Build history of the part. All positions in model axes, mm. A direction names the side the tool comes from. Round coordinates to 2 decimals unless told otherwise and drop trailing zeros. Write each loop counter-clockwise with the first axis right and the second up, starting at its lowest first coordinate (ties: lowest second). Pieces come first, ordered by that corner, then holes. Notation, with made-up numbers: M -14,-23 L 7,-23 A20 cw 7,16 Z; hole C 82,19 d3. An arc over 180 degrees is marked long. Use a Markdown table: item, result.
Autodesk Inventor part; units mm, degrees
ref_plane "XZ Plane" through (0, 0, 0) normal (0, 1, 0) x (-1, 0, 0)
ref_plane "XY Plane" through (0, 0, 0) normal (0, 0, 1) x (1, 0, 0)
sketch "Sketch1" plane through (0, 0, 0) normal (0, 0, 1) x (1, 0, 0)
  line L0 (-4, 0) -> (-4, 7)
  line L1 (-4, 7) -> (-4.5, 7.5)
  line L2 (-4.5, 7.5) -> (-4.5, 48.5)
  line L3 (-4.5, 48.5) -> (-33, 48.5)
  line L4 (-33, 48.5) -> (-33, 49)
  line L5 (-33, 49) -> (-39, 49)
  line L6 (-33.5, 44) -> (-11, 44)
  line L7 (-11, 44) -> (-11, 3)
  line L8 (-11, 3) -> (-8, 0)
  line L9 (-8, 0) -> (-4, 0)
  line L10 (0, 0) -> (0, 13.1371)
  line L11 (-39, 49) -> (-39, -4.5)
  line L12 (-39, -4.5) -> (-34.5, -4.5)
  line L13 (-34.5, -4.5) -> (-34.5, -5.5)
  line L14 (-34.5, -5.5) -> (-33.5, -5.5)
  line L15 (-33.5, -5.5) -> (-33.5, 44)
  line L16 (-33, 48.5) -> (-33, 48.25)
  line L17 (-33, 48.25) -> (-31.5, 48.5)
  line L18 (-35, -4.5) -> (-34.5, -4.35)
  line L19 (-34.5, -4.35) -> (-34.5, -4.5)
  dimension "d0" = 8
  dimension "d1" = 7
  dimension "d7" = 135
  dimension "d9" = 135
  dimension "d11" = 4.5
  dimension "d12" = 9
  dimension "d13" = 16
  dimension "d14" = 22
  dimension "d15" = 0.5
  dimension "d19" = 44
  dimension "d20" = 66
  dimension "d27" = 6.5
  dimension "d28" = 49
  dimension "d29" = 5
  dimension "d31" = 67
  dimension "d32" = 4.5
  dimension "d34" = 1
  dimension "d35" = 0.25
  dimension "d36" = 1.5
  dimension "d37" = 78
  dimension "d38" = 5.5
  dimension "d39" = 0.15
  dimension "d40" = 0.5
  dimension "d41" = 4.5
revolve "Revolution1" add sketch "Sketch1" angle 360 about axis through (0, 0, 0) along (0, 1, 0) contours L9 L8 L7 L6 L15 L14 L13 L19 L18 L12 L11 L5 L4 L16 L17 L3 L2 L1 L0
chamfer "Chamfer1" distance 1 angle 45 1 edges at (4.5, 48.5, 0)
ref_plane "Work Plane1" through (-39, 22.25, 0) normal (1, 0, 0) x (0, 1, 0)
sketch "Sketch2" plane through (-39, 22.25, 0) normal (1, 0, 0) x (0, 1, 0)
  line L0 (-22.75, 0) -> (-37.8891, 0) construction
  line L1 (-22.75, 3) -> (-37.8891, 3)
  line L2 (-37.8891, -3) -> (-22.75, -3)
  arc A0 (-22.75, -3) -> (-22.75, 3) centre (-22.75, 0) ccw
  arc A1 (-37.8891, 3) -> (-37.8891, -3) centre (-37.8891, 0) ccw
  line L3 (-27.75, -34.5) -> (-27.75, 34.5)
  point P0 (-22.25, 0)
  point P1 (-30.3196, 0)
  dimension "d42" = 6
  dimension "d43" = 5
extrude "Extrusion1" cut sketch "Sketch2" along normal blind 10
chamfer "Chamfer2" distance 1 angle 45 1 edges at (39, 49, 0)
properties part number "010" material "Stainless Steel, 440C"
Q1. Drop flat-ended pins along their axis: P1, Ø1, axis at x = -25.5, y = 0.5, coming from the +Z side; P2, Ø8, axis at x = 4, z = -1.5, coming from the -Y side; P3, Ø10, axis at y = 28, z = -19.5, coming from the +X side. Give the stop position or say it passes through.
Response values:
| item | result |
|---|---|
| P1 | stops at z = 29.93 |
| P2 | stops at y = 0 |
| P3 | stops at x = 36.2 |
Q2. Which spindle directions (+Z, -Z, +X, -X, +Y, -Y) get a long thin tool onto all of the face, cutting with end or side? Do faces 4 (the cylindrical face through (2.38, 23.21, 10.74)), 5 (the cylindrical face through (0.867, 3.549, -3.905)), 6 (the flat face through (-7, 48.5, 0)), 7 (the flat face through (-33, -5.5, -8)), 8 (the cylindrical face through (-36.2, 2.5, 0.1)). Say none if no direction does.
Response values:
| item | result |
|---|---|
| face 4 | -Y |
| face 5 | +Y, -Y |
| face 6 | +Y |
| face 7 | +Z, -Z, +X, -X, -Y |
| face 8 | -X, -Y |
Q3. Drill centre lines: L1, parallel to Z at x = 0, y = 35.5; L2, parallel to X at y = 42, z = -6; L3, parallel to X at y = 45, z = 2.5. Where is each one in solid material? Low to high.
Response values:
| item | result |
|---|---|
| L1 | z = -39 to -33.5, -11 to -4.5, 4.5 to 11, 33.5 to 39 |
| L2 | x = -38.54 to -32.96, -9.22 to 9.22, 32.96 to 38.54 |
| L3 | x = -38.92 to -3.74, 3.74 to 38.92 |
Q4. Cut at A-A on y = 42.5. Give the cut face in (x, z), and give its area (3 significant figures).
Response values:
| item | result |
|---|---|
| outline | C 0,0 d78; C 0,0 d22; hole C 0,0 d67; hole C 0,0 d9 |
| area | 1,570 mm2 |
Q5. Two-plate mould, pull along X, no slides. Class faces 1 (the cylindrical face through (5.077, 21.382, -38.668)), 2 (the flat face through (32, -4.5, 15)), 3 (the cylindrical face through (0.59, 27.78, 4.46)): +X half, -X half, draft (parallel to the pull), parting line (faces both ways), or undercut.
Response values:
| item | result |
|---|---|
| face 1 | parting line |
| face 2 | draft |
| face 3 | undercut |
